```python
from build123d import *

# Parameters (mm, degrees)
CROQUIS1_W                                           = 85
CROQUIS1_H                                           = 30
EXTRUIR1_DEPTH                                       = 8
CROQUIS2_W                                           = 8
CROQUIS2_H                                           = 30
EXTRUIR2_DEPTH                                       = 30
CROQUIS3_W                                           = 72.5
CROQUIS3_H                                           = 12
EXTRUIR3_DEPTH                                       = 17.5
CROQUIS4_W                                           = 5
CROQUIS4_H                                           = 8
CORTAR_EXTRUIR1_DEPTH                                = 72.5
CHAFL_N1_SIZE                                        = 5
CROQUIS5_R                                           = 4
CORTAR_EXTRUIR2_DEPTH                                = 20
CHAFL_N2_SIZE                                        = 0.75
REFRENTADO_PARA_TORNILLO_DE_CABEZA_ALLEN_D           = 3.5
REFRENTADO_PARA_TORNILLO_DE_CABEZA_ALLEN_CBORE_D     = 7
REFRENTADO_PARA_TORNILLO_DE_CABEZA_ALLEN_CBORE_DEPTH = 3
CHAFL_N3_SIZE                                        = 0.25
CROQUIS9_W                                           = 6
CROQUIS9_H                                           = 5
SALIENTE_EXTRUIR1_DEPTH                              = 30
CROQUIS10_R                                          = 1.75
CORTAR_EXTRUIR3_DEPTH                                = 5
CROQUIS11_R                                          = 1.75
CORTAR_EXTRUIR4_DEPTH                                = 5


with BuildPart() as part:
    # Croquis1 → Extruir1 (new body)
    with BuildSketch(Plane.XY):
        Rectangle(CROQUIS1_W, CROQUIS1_H)
    extrude(amount=EXTRUIR1_DEPTH)

    # Croquis2 → Extruir2 (add)
    with BuildSketch(Plane.XY.offset(8)):
        with Locations((-38.5, 0)):
            Rectangle(CROQUIS2_W, CROQUIS2_H)
    extrude(amount=EXTRUIR2_DEPTH)

    # Croquis3 → Extruir3 (add)
    with BuildSketch(Plane.XY.offset(8)):
        with Locations((6.25, 0)):
            Rectangle(CROQUIS3_W, CROQUIS3_H)
    extrude(amount=EXTRUIR3_DEPTH)

    # Croquis4 → Cortar-Extruir1 (cut)
    with BuildSketch(Plane(origin=(42.5, 0, 0), x_dir=(0, 0, -1), z_dir=(1, 0, 0))):
        with Locations((-23, 0)):
            Rectangle(CROQUIS4_W, CROQUIS4_H)
    extrude(amount=-CORTAR_EXTRUIR1_DEPTH, mode=Mode.SUBTRACT)

    # Chaflán1
    chafl_n1_edges = [part.edges().sort_by_distance(p)[0] for p in [
        (-38.5, -15, 38),
        (-38.5, 15, 38),
    ]]
    chamfer(chafl_n1_edges, length=CHAFL_N1_SIZE)

    # Croquis5 → Cortar-Extruir2 (cut)
    with BuildSketch(Plane(origin=(-34.5, 0, 0), x_dir=(0, 0, -1), z_dir=(1, 0, 0))):
        with Locations(Location((-24.5, 0, 0), (0, 0, 90))):
            Circle(CROQUIS5_R)
    extrude(amount=-CORTAR_EXTRUIR2_DEPTH, mode=Mode.SUBTRACT)

    # Chaflán2
    chafl_n2_edges = [part.edges().sort_by_distance(p)[0] for p in [
        (-42.5, -4, 24.5),
        (-34.5, -4, 24.5),
    ]]
    chamfer(chafl_n2_edges, length=CHAFL_N2_SIZE)

    # Refrentado para tornillo de cabeza allen de M6-1 (through all)
    with Locations(Plane.XY.offset(8)):
        with Locations((-28.5, 10.5), (-28.5, -10.5), (36.5, -10.5), (36.5, 10.5)):
            CounterBoreHole(REFRENTADO_PARA_TORNILLO_DE_CABEZA_ALLEN_D / 2, REFRENTADO_PARA_TORNILLO_DE_CABEZA_ALLEN_CBORE_D / 2, REFRENTADO_PARA_TORNILLO_DE_CABEZA_ALLEN_CBORE_DEPTH)

    # Chaflán3
    chafl_n3_edges = [part.edges().sort_by_distance(p)[0] for p in [
        (-32, 10.5, 8),
        (33, 10.5, 8),
        (33, -10.5, 8),
        (-32, -10.5, 8),
    ]]
    chamfer(chafl_n3_edges, length=CHAFL_N3_SIZE)

    # Croquis9 → Saliente-Extruir1 (add)
    with BuildSketch(Plane.XY.offset(8)):
        with Locations((-20.75, -9.5)):
            Rectangle(CROQUIS9_W, CROQUIS9_H)
        with Locations((28.75, -9.5)):
            Rectangle(CROQUIS9_W, CROQUIS9_H)
    extrude(amount=SALIENTE_EXTRUIR1_DEPTH)

    # Croquis10 → Cortar-Extruir3 (cut)
    with BuildSketch(Plane(origin=(0, -7, 0), x_dir=(1, 0, 0), z_dir=(0, 1, 0))):
        with Locations(Location((-20.75, -32.38, 0), (0, 0, 270))):
            Circle(CROQUIS10_R)
    extrude(amount=-CORTAR_EXTRUIR3_DEPTH, mode=Mode.SUBTRACT)

    # Croquis11 → Cortar-Extruir4 (cut)
    with BuildSketch(Plane(origin=(0, -7, 0), x_dir=(1, 0, 0), z_dir=(0, 1, 0))):
        with Locations(Location((28.75, -32.38, 0), (0, 0, 270))):
            Circle(CROQUIS11_R)
    extrude(amount=-CORTAR_EXTRUIR4_DEPTH, mode=Mode.SUBTRACT)


solid = part.part
```
The model under review builds one solid part; all positions refer to its coordinate system, in mm. A direction names the side the tool comes from. Round coordinates to 2 decimals unless told otherwise and drop trailing zeros. Order: outer loops, then holes, each group sorted by start corner. A loop starts at its lowest first (then second) coordinate and runs counter-clockwise, first axis right, second up. Notation, with made-up numbers: (31, 74) -> (70, 74) arc R32 cw to (70, 108) -> close; hole circle Ø4 at (1, 6.5). An arc over 180 degrees is marked (long way). One line per item, written item: value. Start each with the question number.
Q1. Machinability: for faces 4 (the face through (38, 9, 5)), 5 (the face through (6, 6, 17)), 6 (the face through (-17.75, -10, 23)), 7 (the face through (-21, -7, 23)), which of the approach directions +Z, -Z, +X, -X, +Y, -Y give a long, thin tool a straight path to every point of the face, cutting with its end or side? Answer none if there is none.
Q2. Take a section at D-D (x = 19). Write out the cut boundary in (y, z).
Q3. Take a section at A-A (z = 17). Write out the cut boundary in (x, y).
Q4. Take a section at C-C (z = 24.5). Write out the cut boundary in (x, y).
Q5. Take a section at B-B (x = -20.75). Write out the cut boundary in (y, z), and give its area (4 significant figures).
Q6. Wall thickness on line 1 (Y direction, x = 36.5, z = 6.45); line 2 (X direction, y = -10.2, z = 32.38); line 3 (X direction, y = -10.75, z = 29.5): over which ranges is each line inside the solid? List them lowest first.
Q7. Clearance check with flat-ended pins moving along their axes: pin 1 Ø4 at (y, z) = (-9, 20) entering from +X; pin 2 Ø3.5 at (x, y) = (35.5, -11.5) entering from +Z; pin 3 Ø3 at (x, z) = (33, 17) entering from +Y; pin 4 Ø6.5 at (y, z) = (0, 24.5) entering from +X. State where each tip first meets the part, or that it passes through.
Q8. Mouldability with a two-part tool opening along Y and no side actions: class faces 1 (the face through (-39, -13, 35)), 2 (the face through (-38.454, -0.521, 28.466)), 3 (the face through (28.08, -9.465, 33.997)) as released by +Y, released by -Y, zero draft, split by the parting line, or undercut.
Reported:
1. face 4: +Z
1. face 5: +Z, +X, +Y
1. face 6: +Z, -Y
1. face 7: +Z, +X
2. outline: (-15, 0) -> (15, 0) -> (15, 8) -> (6, 8) -> (6, 25.5) -> (4, 25.5) -> (4, 20.5) -> (-4, 20.5) -> (-4, 25.5) -> (-6, 25.5) -> (-6, 8) -> (-15, 8) -> close
3. outline: (-42.5, -15) -> (-34.5, -15) -> (-34.5, 15) -> (-42.5, 15) -> close; (-30, -6) -> (42.5, -6) -> (42.5, 6) -> (-30, 6) -> close; (-23.75, -12) -> (-17.75, -12) -> (-17.75, -7) -> (-23.75, -7) -> close; (25.75, -12) -> (31.75, -12) -> (31.75, -7) -> (25.75, -7) -> close
4. outline: (-42.5, -15) -> (-34.5, -15) -> (-34.5, -4.75) -> (-35.25, -4) -> (-41.75, -4) -> (-42.5, -4.75) -> close; (-42.5, 4.75) -> (-41.75, 4) -> (-35.25, 4) -> (-34.5, 4.75) -> (-34.5, 15) -> (-42.5, 15) -> close; (-30, -6) -> (42.5, -6) -> (42.5, -4) -> (-30, -4) -> close; (-30, 4) -> (42.5, 4) -> (42.5, 6) -> (-30, 6) -> close; (-23.75, -12) -> (-17.75, -12) -> (-17.75, -7) -> (-23.75, -7) -> close; (25.75, -12) -> (31.75, -12) -> (31.75, -7) -> (25.75, -7) -> close
5. outline: (-15, 0) -> (15, 0) -> (15, 8) -> (6, 8) -> (6, 25.5) -> (4, 25.5) -> (4, 20.5) -> (-4, 20.5) -> (-4, 25.5) -> (-6, 25.5) -> (-6, 8) -> (-7, 8) -> (-7, 30.63) -> (-12, 30.63) -> (-12, 8) -> (-15, 8) -> close; (-12, 34.13) -> (-7, 34.13) -> (-7, 38) -> (-12, 38) -> close
5. area: 542.5 mm2
6. line 1: y = -15 to -14, -7 to 7, 14 to 15
6. line 2: x = -42.5 to -34.5, -23.75 to -22.5, -19 to -17.75, 25.75 to 27, 30.5 to 31.75
6. line 3: x = -42.5 to -34.5, -23.75 to -17.75, 25.75 to 31.75
7. pin 1: stops at x = 31.75
7. pin 2: stops at z = 5
7. pin 3: stops at y = 6
7. pin 4: passes through
8. face 1: released by -Y
8. face 2: undercut
8. face 3: zero draft
